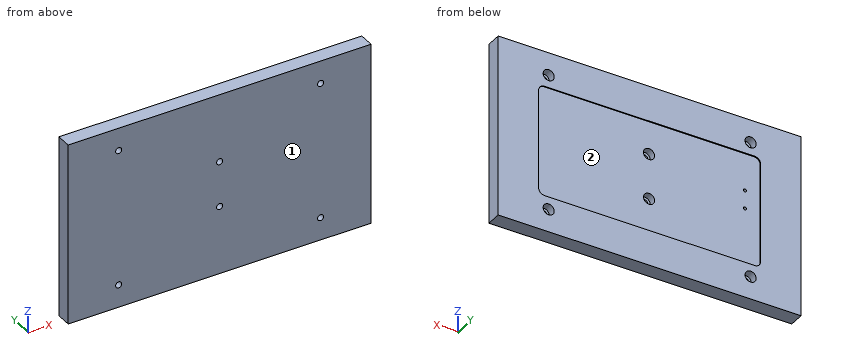
from build123d import *

# Parameters (mm, degrees)
SKETCH_1_W          = 300
SKETCH_1_H          = 180
EXTRUDE_1_DEPTH     = 15
SKETCH_2_R          = 3
SKETCH_2_R_2        = 2.5
CUT_EXTRUDE_1_DEPTH = 176.570498661
SKETCH_3_R          = 5.5
SKETCH_3_R_2        = 5
SKETCH_3_R_3        = 3
CUT_EXTRUDE_3_DEPTH = 8
CUT_EXTRUDE_4_DEPTH = 1
CUT_EXTRUDE_START   = -9
SKETCH_6_R          = 1.55
CUT_EXTRUDE_6_DEPTH = 9


with BuildPart() as part:
    # Эскиз1 → Бобышка-Вытянуть1 (new body)
    with BuildSketch(Plane(origin=(0, 0, 0), x_dir=(1, 0, 0), z_dir=(0, 1, 0))):
        Rectangle(SKETCH_1_W, SKETCH_1_H)
    extrude(amount=EXTRUDE_1_DEPTH)

    # Эскиз2 → Вырез-Вытянуть1 (cut, through all)
    # profile 1 of 12: a face of its own
    with BuildSketch(Plane(origin=(0, 15, 0), x_dir=(1, 0, 0), z_dir=(0, 1, 0))):
        with Locations(Location((0, -22.5, 0), (0, 0, 270))):
            Circle(SKETCH_2_R)
        with Locations((0, -22.5)):
            Circle(SKETCH_2_R_2, mode=Mode.SUBTRACT)
    # profile 2 of 12: a face of its own
    with BuildSketch(Plane(origin=(0, 15, 0), x_dir=(1, 0, 0), z_dir=(0, 1, 0))):
        with Locations((0, -22.5)):
            Circle(SKETCH_2_R_2)
    # profile 3 of 12: a face of its own
    with BuildSketch(Plane(origin=(0, 15, 0), x_dir=(1, 0, 0), z_dir=(0, 1, 0))):
        with Locations(Location((-100, -67.5, 0), (0, 0, 270))):
            Circle(SKETCH_2_R)
        with Locations((-100, -67.5)):
            Circle(SKETCH_2_R_2, mode=Mode.SUBTRACT)
    # profile 4 of 12: a face of its own
    with BuildSketch(Plane(origin=(0, 15, 0), x_dir=(1, 0, 0), z_dir=(0, 1, 0))):
        with Locations((-100, -67.5)):
            Circle(SKETCH_2_R_2)
    # profile 5 of 12: a face of its own
    with BuildSketch(Plane(origin=(0, 15, 0), x_dir=(1, 0, 0), z_dir=(0, 1, 0))):
        with Locations(Location((100, -67.5, 0), (0, 0, 270))):
            Circle(SKETCH_2_R)
        with Locations((100, -67.5)):
            Circle(SKETCH_2_R_2, mode=Mode.SUBTRACT)
    # profile 6 of 12: a face of its own
    with BuildSketch(Plane(origin=(0, 15, 0), x_dir=(1, 0, 0), z_dir=(0, 1, 0))):
        with Locations((100, -67.5)):
            Circle(SKETCH_2_R_2)
    # profile 7 of 12: a face of its own
    with BuildSketch(Plane(origin=(0, 15, 0), x_dir=(1, 0, 0), z_dir=(0, 1, 0))):
        with Locations(Location((100, 67.5, 0), (0, 0, 270))):
            Circle(SKETCH_2_R)
        with Locations((100, 67.5)):
            Circle(SKETCH_2_R_2, mode=Mode.SUBTRACT)
    # profile 8 of 12: a face of its own
    with BuildSketch(Plane(origin=(0, 15, 0), x_dir=(1, 0, 0), z_dir=(0, 1, 0))):
        with Locations((100, 67.5)):
            Circle(SKETCH_2_R_2)
    # profile 9 of 12: a face of its own
    with BuildSketch(Plane(origin=(0, 15, 0), x_dir=(1, 0, 0), z_dir=(0, 1, 0))):
        with Locations(Location((0, 22.5, 0), (0, 0, 270))):
            Circle(SKETCH_2_R)
        with Locations((0, 22.5)):
            Circle(SKETCH_2_R_2, mode=Mode.SUBTRACT)
    # profile 10 of 12: a face of its own
    with BuildSketch(Plane(origin=(0, 15, 0), x_dir=(1, 0, 0), z_dir=(0, 1, 0))):
        with Locations((0, 22.5)):
            Circle(SKETCH_2_R_2)
    # profile 11 of 12: a face of its own
    with BuildSketch(Plane(origin=(0, 15, 0), x_dir=(1, 0, 0), z_dir=(0, 1, 0))):
        with Locations(Location((-100, 67.5, 0), (0, 0, 270))):
            Circle(SKETCH_2_R)
        with Locations((-100, 67.5)):
            Circle(SKETCH_2_R_2, mode=Mode.SUBTRACT)
    # profile 12 of 12: a face of its own
    with BuildSketch(Plane(origin=(0, 15, 0), x_dir=(1, 0, 0), z_dir=(0, 1, 0))):
        with Locations((-100, 67.5)):
            Circle(SKETCH_2_R_2)
    extrude(amount=-CUT_EXTRUDE_1_DEPTH, mode=Mode.SUBTRACT)

    # Эскиз3 → Вырез-Вытянуть3 (cut)
    # profile 1 of 12: a face of its own
    with BuildSketch(Plane(origin=(0, 15, 0), x_dir=(1, 0, 0), z_dir=(0, 1, 0))):
        with Locations(Location((0, -22.5, 0), (0, 0, 270))):
            Circle(SKETCH_3_R)
        with Locations((0, -22.5)):
            Circle(SKETCH_3_R_2, mode=Mode.SUBTRACT)
    # profile 2 of 12: a face of its own
    with BuildSketch(Plane(origin=(0, 15, 0), x_dir=(1, 0, 0), z_dir=(0, 1, 0))):
        with Locations((0, -22.5)):
            Circle(SKETCH_3_R_2)
        with Locations(Location((0, -22.5, 0), (0, 0, 270))):
            Circle(SKETCH_3_R_3, mode=Mode.SUBTRACT)
    # profile 3 of 12: a face of its own
    with BuildSketch(Plane(origin=(0, 15, 0), x_dir=(1, 0, 0), z_dir=(0, 1, 0))):
        with Locations(Location((-100, -67.5, 0), (0, 0, 270))):
            Circle(SKETCH_3_R)
        with Locations((-100, -67.5)):
            Circle(SKETCH_3_R_2, mode=Mode.SUBTRACT)
    # profile 4 of 12: a face of its own
    with BuildSketch(Plane(origin=(0, 15, 0), x_dir=(1, 0, 0), z_dir=(0, 1, 0))):
        with Locations((-100, -67.5)):
            Circle(SKETCH_3_R_2)
        with Locations(Location((-100, -67.5, 0), (0, 0, 270))):
            Circle(SKETCH_3_R_3, mode=Mode.SUBTRACT)
    # profile 5 of 12: a face of its own
    with BuildSketch(Plane(origin=(0, 15, 0), x_dir=(1, 0, 0), z_dir=(0, 1, 0))):
        with Locations(Location((100, -67.5, 0), (0, 0, 270))):
            Circle(SKETCH_3_R)
        with Locations((100, -67.5)):
            Circle(SKETCH_3_R_2, mode=Mode.SUBTRACT)
    # profile 6 of 12: a face of its own
    with BuildSketch(Plane(origin=(0, 15, 0), x_dir=(1, 0, 0), z_dir=(0, 1, 0))):
        with Locations((100, -67.5)):
            Circle(SKETCH_3_R_2)
        with Locations(Location((100, -67.5, 0), (0, 0, 270))):
            Circle(SKETCH_3_R_3, mode=Mode.SUBTRACT)
    # profile 7 of 12: a face of its own
    with BuildSketch(Plane(origin=(0, 15, 0), x_dir=(1, 0, 0), z_dir=(0, 1, 0))):
        with Locations(Location((0, 22.5, 0), (0, 0, 270))):
            Circle(SKETCH_3_R)
        with Locations((0, 22.5)):
            Circle(SKETCH_3_R_2, mode=Mode.SUBTRACT)
    # profile 8 of 12: a face of its own
    with BuildSketch(Plane(origin=(0, 15, 0), x_dir=(1, 0, 0), z_dir=(0, 1, 0))):
        with Locations((0, 22.5)):
            Circle(SKETCH_3_R_2)
        with Locations(Location((0, 22.5, 0), (0, 0, 270))):
            Circle(SKETCH_3_R_3, mode=Mode.SUBTRACT)
    # profile 9 of 12: a face of its own
    with BuildSketch(Plane(origin=(0, 15, 0), x_dir=(1, 0, 0), z_dir=(0, 1, 0))):
        with Locations(Location((-100, 67.5, 0), (0, 0, 270))):
            Circle(SKETCH_3_R)
        with Locations((-100, 67.5)):
            Circle(SKETCH_3_R_2, mode=Mode.SUBTRACT)
    # profile 10 of 12: a face of its own
    with BuildSketch(Plane(origin=(0, 15, 0), x_dir=(1, 0, 0), z_dir=(0, 1, 0))):
        with Locations((-100, 67.5)):
            Circle(SKETCH_3_R_2)
        with Locations(Location((-100, 67.5, 0), (0, 0, 270))):
            Circle(SKETCH_3_R_3, mode=Mode.SUBTRACT)
    # profile 11 of 12: a face of its own
    with BuildSketch(Plane(origin=(0, 15, 0), x_dir=(1, 0, 0), z_dir=(0, 1, 0))):
        with Locations(Location((100, 67.5, 0), (0, 0, 270))):
            Circle(SKETCH_3_R)
        with Locations((100, 67.5)):
            Circle(SKETCH_3_R_2, mode=Mode.SUBTRACT)
    # profile 12 of 12: a face of its own
    with BuildSketch(Plane(origin=(0, 15, 0), x_dir=(1, 0, 0), z_dir=(0, 1, 0))):
        with Locations((100, 67.5)):
            Circle(SKETCH_3_R_2)
        with Locations(Location((100, 67.5, 0), (0, 0, 270))):
            Circle(SKETCH_3_R_3, mode=Mode.SUBTRACT)
    extrude(amount=-CUT_EXTRUDE_3_DEPTH, mode=Mode.SUBTRACT)

    # Эскиз4 → Вырез-Вытянуть4 (cut)
    with BuildSketch(Plane(origin=(0, 15, 0), x_dir=(1, 0, 0), z_dir=(0, 1, 0))):
        with BuildLine():
            Line((-110, -49), (-110, 49))
            ThreePointArc((-110, 49), (-108.242640687, 53.242640687), (-104, 55))
            Line((-104, 55), (104, 55))
            ThreePointArc((104, 55), (108.242640687, 53.242640687), (110, 49))
            Line((110, 49), (110, -49))
            ThreePointArc((110, -49), (108.242640687, -53.242640687), (104, -55))
            Line((104, -55), (-104, -55))
            ThreePointArc((-104, -55), (-108.242640687, -53.242640687), (-110, -49))
        make_face()
    extrude(amount=-CUT_EXTRUDE_4_DEPTH, mode=Mode.SUBTRACT)

    # Эскиз6 → Вырез-Вытянуть6 (cut)
    with BuildSketch(Plane(origin=(0, 14, 0), x_dir=(1, 0, 0), z_dir=(0, 1, 0)).offset(CUT_EXTRUDE_START)):
        with Locations(Location((-95, -18, 0), (0, 0, 270))):
            Circle(SKETCH_6_R)
        with Locations(Location((-95, 0, 0), (0, 0, 270))):
            Circle(SKETCH_6_R)
    extrude(amount=CUT_EXTRUDE_6_DEPTH, mode=Mode.SUBTRACT)


solid = part.part
Build history of the part. All positions in model axes, mm. Face numbers are marked on the shaded views. Coordinates: 2 decimals unless noted, no trailing zeros. Write each loop counter-clockwise with the first axis right and the second up, starting at its lowest first coordinate (ties: lowest second). Pieces come first, ordered by that corner, then holes. Notation, with made-up numbers: (12.25, 49) -> (62.25, 49) arc R12 ccw to (62.25, 62) -> close; hole circle Ø8 at (12, -14.75). An arc over 180 degrees is marked (long way). Use CSV: the item, a comma, the result in double quotes. Start each with the question number.
Q1. Cut at C-C, the plane z = 67.5. List the corners of the cut face in (x, y).
Q2. Cut at B-B, the plane x = -100. List the corners of the cut face in (y, z), then the cut area to 3 significant figures.
Q3. Cut at D-D, the plane x = 50.5. List the corners of the cut face in (y, z).
Q4. Cut at A-A, the plane z = -22.5. List the corners of the cut face in (x, y), then the cut area to 3 significant figures.
Q5. Pull direction X, two halves, no side cores. Call the marked faces 1 and 2: released by +X, released by -X, zero draft, split by the parting line, or undercut.
Q6. Flat gauge pins, fed straight in: pin 1 Ø8 at (x, z) = (100, -67.5) entering from +Y; pin 2 Ø1 at (x, z) = (-93, -40) entering from +Y. Where does each tip first touch, or does it go through?
Q7. Drill centre lines: probe 1 along X at (y, z) = (9.5, -67.5); probe 2 along X at (y, z) = (4, -67.5); probe 3 along Y at (x, z) = (-96, -40). Where is each one in solid material? Low to high.
Checked values:
1,outline,"(-150, 0) -> (-103, 0) -> (-103, 7) -> (-105.5, 7) -> (-105.5, 15) -> (-150, 15) -> close; (-97, 0) -> (97, 0) -> (97, 7) -> (94.5, 7) -> (94.5, 15) -> (-94.5, 15) -> (-94.5, 7) -> (-97, 7) -> close; (103, 0) -> (150, 0) -> (150, 15) -> (105.5, 15) -> (105.5, 7) -> (103, 7) -> close"
2,outline,"(0, -90) -> (15, -90) -> (15, -73) -> (7, -73) -> (7, -70.5) -> (0, -70.5) -> close; (0, -64.5) -> (7, -64.5) -> (7, -62) -> (15, -62) -> (15, -55) -> (14, -55) -> (14, 55) -> (15, 55) -> (15, 62) -> (7, 62) -> (7, 64.5) -> (0, 64.5) -> close; (0, 70.5) -> (7, 70.5) -> (7, 73) -> (15, 73) -> (15, 90) -> (0, 90) -> close"
2,area,"2,330 mm²"
3,outline,"(0, -90) -> (15, -90) -> (15, -55) -> (14, -55) -> (14, 55) -> (15, 55) -> (15, 90) -> (0, 90) -> close"
4,outline,"(-150, 0) -> (-3, 0) -> (-3, 7) -> (-5.5, 7) -> (-5.5, 14) -> (-110, 14) -> (-110, 15) -> (-150, 15) -> close; (3, 0) -> (150, 0) -> (150, 15) -> (110, 15) -> (110, 14) -> (5.5, 14) -> (5.5, 7) -> (3, 7) -> close"
4,area,"4,160 mm²"
5,face 1,"zero draft"
5,face 2,"undercut"
6,pin 1,"stops at y = 7"
6,pin 2,"stops at y = 14"
7,probe 1,"x = -150 to -105.5, -94.5 to 94.5, 105.5 to 150"
7,probe 2,"x = -150 to -103, -97 to 97, 103 to 150"
7,probe 3,"y = 0 to 14"
